Here's how the part is built. I have some questions about the finished solid (model axes, mm). A direction names the side the tool comes from. Give positions to 0.01 mm unless a question says otherwise; leave off trailing zeros. Write each loop counter-clockwise with the first axis right and the second up, starting at its lowest first coordinate (ties: lowest second). Pieces come first, ordered by that corner, then holes. Notation, with made-up numbers: (-21, 56.25) - (10, 56.25) arc R16 cw to (10, 63.25) - close; hole circle Ø2 at (-40, 58.25). An arc over 180 degrees is marked (long way). One line per item, written item: value. Start each with the question number.
1) Imagine slicing it at A-A on x = 0. Write out the boundary of the cut face in (y, z) (1 decimal).
2) We'd pull the mould along X, two halves only. Please class faces 3 (the flat face through (-6, -31.75, 2)), 4 (the cylindrical face through (-4.3, -4.95, 2.35)), 5 (the flat face through (-9.525, -16, 2)): +X half, -X half, draft (parallel to the pull), parting line (faces both ways), or undercut.
3) Imagine slicing it at C-C on z = 3.25. Count the separate pieces of the cut face and the enclosed holes in it, plus the area to 3 significant figures.
4) Imagine slicing it at D-D on y = 7. Write out the boundary of the cut face in (x, z), plus the area to 3 significant figures.
5) On a 3-axis mill with a long thin cutter (end or side, diameter ignored), from which of +Z, -Z, +X, -X, +Y, -Y can I reach the whole of each face in a straight line? I mean faces 1 (the flat face through (9.525, -16, 2)), 2 (the flat face through (-1.588, -23, 2)). Say none if no direction works.
6) Please list where these lines run through material, in increasing order: L1, parallel to X at y = -20, z = 3.15 (1 decimal); L2, parallel to Y at x = 2, z = 3.3; L3, parallel to Y at x = -7.5, z = 3.8. Write a range as [from, to].
7) Imagine slicing it at B-B on y = -25. Write out the boundary of the cut face in (x, z) (1 decimal), plus the area to 3 significant figures.
from build123d import *

# Parameters (mm, degrees)
F0_R     = 0.5
F0_R_2   = 2.5
F1_DEPTH = 4.7625


with BuildPart() as f1:
    # F0 (on Top) → F1 (new body)
    with BuildSketch(Plane.XY):
        with BuildLine():
            Line((9.525, -31.75), (9.525, 0))
            ThreePointArc((9.525, 0), (0, 9.525), (-9.525, 0))
            Line((-9.525, 0), (-9.525, -31.75))
            Line((-9.525, -31.75), (-1.5875, -31.75))
            Line((-1.5875, -31.75), (-1.5875, -14.2875))
            Line((-1.5875, -14.2875), (1.5875, -14.2875))
            Line((1.5875, -14.2875), (1.5875, -31.75))
            Line((1.5875, -31.75), (9.525, -31.75))
        make_face()
        with Locations((-4.7625, -4.7625)):
            Circle(F0_R, mode=Mode.SUBTRACT)
        with Locations((4.7625, -4.7625)):
            Circle(F0_R, mode=Mode.SUBTRACT)
        Circle(F0_R_2, mode=Mode.SUBTRACT)
    extrude(amount=F1_DEPTH)


solid = f1.part
Numbers:
1. outline: (-14.3, 0) - (-2.5, 0) - (-2.5, 4.8) - (-14.3, 4.8) - close; (2.5, 0) - (9.5, 0) - (9.5, 4.8) - (2.5, 4.8) - close
2. face 3: draft
2. face 4: undercut
2. face 5: -X half
3. separate pieces: 1
3. enclosed holes: 3
3. area: 671 mm^2
4. outline: (-6.46, 0) - (6.46, 0) - (6.46, 4.76) - (-6.46, 4.76) - close
4. area: 61.5 mm^2
5. face 1: +Z, -Z, +X, +Y, -Y
5. face 2: +Z, -Z, -Y
6. L1: [-9.5, -1.6], [1.6, 9.5]
6. L2: [-31.75, -1.5], [1.5, 9.31]
6. L3: [-31.75, 5.87]
7. outline: (-9.5, 0) - (-1.6, 0) - (-1.6, 4.8) - (-9.5, 4.8) - close; (1.6, 0) - (9.5, 0) - (9.5, 4.8) - (1.6, 4.8) - close
7. area: 75.6 mm^2
